Autodesk Inventor part; units mm, degrees
ref_plane "YZ Plane" through (0, 0, 0) normal (1, 0, 0) x (0, 1, 0)
ref_plane "XZ Plane" through (0, 0, 0) normal (0, 1, 0) x (-1, 0, 0)
ref_plane "XY Plane" through (0, 0, 0) normal (0, 0, 1) x (1, 0, 0)
sketch "Sketch1" plane through (0, 0, 0) normal (0, 0, 1) x (1, 0, 0)
  line L0 (0, 0) -> (16.764, 0)
  line L1 (16.764, 0) -> (16.764, 25.908)
  line L2 (16.764, 25.908) -> (0, 25.908)
  line L3 (0, 25.908) -> (0, 0)
  dimension "d0" = 16.764
  dimension "d1" = 25.908
extrude "Extrusion1" add sketch "Sketch1" along normal blind 5.334
sketch "Sketch2" plane through (0, 0, 5.334) normal (0, 0, 1) x (1, 0, 0)
  line L0 (-1.524, 29.718) -> (18.288, 29.718)
  line L1 (18.288, 29.718) -> (18.288, -3.81)
  line L2 (18.288, -3.81) -> (-1.524, -3.81)
  line L3 (-1.524, -3.81) -> (-1.524, 29.718)
  line L4 (16.764, 25.908) -> (0, 25.908)
  line L5 (0, 0) -> (16.764, 0)
  line L6 (0, 25.908) -> (0, 0)
  line L7 (16.764, 0) -> (16.764, 25.908)
  dimension "d4" = 3.81
  dimension "d5" = 3.81
  dimension "d6" = 1.524
  dimension "d7" = 1.524
extrude "Extrusion2" add sketch "Sketch2" along normal blind 2.286 contours L0 L1 L2 L3 | L7 L5 L6 L4
sketch "Sketch3" plane through (0, 0, 7.62) normal (0, 0, 1) x (1, 0, 0)
  circle A0 centre (8.382, 12.954) radius 4.826
  line L0 (18.288, 29.718) -> (-1.524, 29.718)
  line L1 (-1.524, -3.81) -> (18.288, -3.81)
  line L2 (-1.524, 29.718) -> (-1.524, -3.81)
  line L3 (18.288, -3.81) -> (18.288, 29.718)
  point P0 (0, 0)
  dimension "d10" = 16.764
  dimension "d11" = 16.764
  dimension "d12" = 9.906
  dimension "d13" = 9.906
  dimension "d14" = 9.652
extrude "Extrusion3" add sketch "Sketch3" along normal blind 27.94 contours A0
sketch "Sketch4" plane through (8.382, 12.954, 35.56) normal (0, 0, 1) x (1, 0, 0)
  circle A0 centre (0, 0) radius 2.413
  line L0 (-0.889, 3.302) -> (0.889, 3.302)
  line L1 (0.889, 3.302) -> (0.889, -3.302)
  line L2 (0.889, -3.302) -> (-0.889, -3.302)
  line L3 (-0.889, -3.302) -> (-0.889, 3.302)
  circle A1 centre (0, 0) radius 4.826
  point P0 (-8.382, -12.954)
  point P1 (-0.889, 0)
  point P2 (0.889, 0)
  point P3 (-0.889, -2.2433)
  point P4 (0.889, -2.2433)
  point P5 (0.889, 2.2433)
  point P6 (-0.889, 2.2433)
  dimension "d17" = 4.826
  dimension "d18" = 0.889
  dimension "d19" = 0.889
  dimension "d20" = 3.302
  dimension "d21" = 3.302
extrude "Extrusion4" cut sketch "Sketch4" against normal blind 27.94 contours A0 L1 | L1 A0 L3 | A0 L3 L0 L1 | L1 L2 L3 A0 | L3 A0
sketch "Sketch5" plane through (0, 0, 0) normal (0, 0, -1) x (-1, 0, 0)
  arc A0 (-7.493, 10.7107) -> (-7.493, 15.1973) centre (-8.382, 12.954) ccw
  circle A1 centre (-8.382, 12.954) radius 6.0325
  point P0 (0, 0)
  dimension "d24" = 12.065
extrude "Extrusion5" cut sketch "Sketch5" against normal blind 1.5875
fillet "Fillet1" radius 3.175 1 edges at (14.4145, 12.954, 1.5875)
fillet "Fillet3" radius 1.5875 4 edges at (-1.524, 29.718, 6.477) (-1.524, -3.81, 6.477) (18.288, 29.718, 6.477) (18.288, -3.81, 6.477)
properties part number "reset_switch"
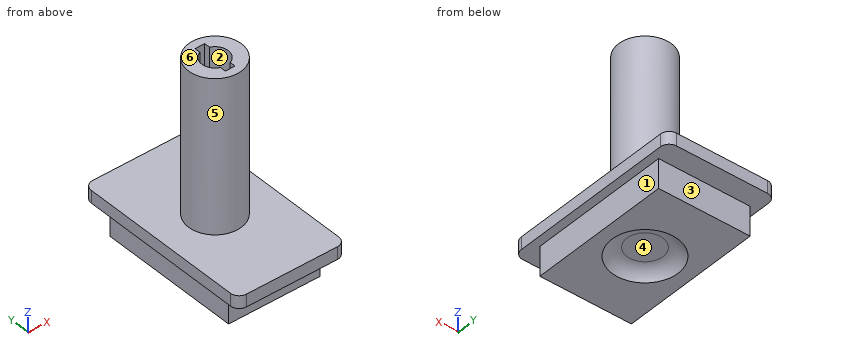
Geometry check sheet. Reference: the model listing, model coordinates, mm. Face numbers are marked on the shaded views. A direction names the side the tool comes from. Give positions to 0.01 mm unless a question says otherwise; leave off trailing zeros. Write each loop counter-clockwise with the first axis right and the second up, starting at its lowest first coordinate (ties: lowest second). Pieces come first, ordered by that corner, then holes.
1) Access from +Z, -Z, +X, -X, +Y, -Y to the whole of each face (thin tool, end or side, straight path). Record for the marked faces 5 and 6.
2) Section check C-C, the plane z = 12.5. Record the boundary of the cut face in (x, y), and give its area (3 significant figures).
3) Section check A-A, the plane y = 22. Record the boundary of the cut face in (x, z).
4) Section check D-D, the plane z = 4.5. Record the boundary of the cut face in (x, y).
5) Material ranges on L1, parallel to Z at x = 15, y = 17.5; L2, parallel to Z at x = 4.75, y = 27; L3, parallel to Y at x = 8.5, z = 14.5, recorded low to high.
6) Release check for a two-part mould opening along X. For the marked faces 1, 2, 3 and 4 record: pulls with the +X half, pulls with the -X half, needs draft (parallel to the pull), parting line crosses it, or undercut.
7) Section check B-B, the plane x = 16.25. Record the boundary of the cut face in (y, z).
8) Gauge pin test, flat ends, axial feed: pin 1 (0.5 mm diameter, centred on y = 10, z = 18, fed in from -X); pin 2 (4 mm diameter, centred on y = 11.5, z = 9, fed in from -X); pin 3 (0.5 mm diameter, centred on y = 16, z = 17.5, fed in from +X); pin 4 (2 mm diameter, centred on x = 9, y = 12.5, fed in from -Z). Record the tip position at first contact, or that the pin passes through.
Computed:
1. face 5: +Z
1. face 6: +Z, +X, -X, +Y, -Y
2. outline: circle Ø9.65 at (8.38, 12.95); hole (7.49, 9.65) - (9.27, 9.65) - (9.27, 10.71) arc R2.41 ccw to (9.27, 15.2) - (9.27, 16.26) - (7.49, 16.26) - (7.49, 15.2) arc R2.41 ccw to (7.49, 10.71) - close
2. area: 51.5 mm2
3. outline: (-1.52, 5.33) - (0, 5.33) - (0, 0) - (16.76, 0) - (16.76, 5.33) - (18.29, 5.33) - (18.29, 7.62) - (-1.52, 7.62) - close
4. outline: (0, 0) - (16.76, 0) - (16.76, 25.91) - (0, 25.91) - close
5. L1: z = 0 to 7.62
5. L2: z = 5.33 to 7.62
5. L3: y = 8.13 to 9.65, 16.26 to 17.78
6. face 1: pulls with the +X half
6. face 2: undercut
6. face 3: needs draft
6. face 4: undercut
7. outline: (-3.81, 5.33) - (0, 5.33) - (0, 0) - (25.91, 0) - (25.91, 5.33) - (29.72, 5.33) - (29.72, 7.62) - (-3.81, 7.62) - close
8. pin 1: stops at x = 4.38
8. pin 2: stops at x = -1.52
8. pin 3: stops at x = 12.32
8. pin 4: stops at z = 1.59
